```python
from build123d import *

# Parameters (mm, degrees)
SKETCH1_W           = 145
SKETCH1_H           = 85
BOSS_EXTRUDE1_DEPTH = 90
SKETCH3_W           = 130
SKETCH3_H           = 80
CUT_EXTRUDE1_DEPTH  = 85
SKETCH8_R           = 1.7
CUT_EXTRUDE2_DEPTH  = 10
SKETCH9_R           = 1.6
CUT_EXTRUDE3_DEPTH  = 10
SKETCH10_W          = 60.36577322
SKETCH10_H          = 26.383642142
CUT_EXTRUDE4_DEPTH  = 176.87282337
SKETCH11_W          = 127.368574342
SKETCH11_H          = 34.248868694
CUT_EXTRUDE5_DEPTH  = 144.461667354
CUT_EXTRUDE8_DEPTH  = 142
SKETCH13_R          = 2.5
CUT_EXTRUDE9_DEPTH  = 10
FILLET1_R           = 5


with BuildPart() as part:
    # Sketch1 → Boss-Extrude1 (new body)
    with BuildSketch(Plane(origin=(0, 0, 0), x_dir=(1, 0, 0), z_dir=(0, 1, 0))):
        Rectangle(SKETCH1_W, SKETCH1_H)
    extrude(amount=BOSS_EXTRUDE1_DEPTH)

    # Sketch3 → Cut-Extrude1 (cut)
    with BuildSketch(Plane(origin=(0, 90, 0), x_dir=(1, 0, 0), z_dir=(0, 1, 0))):
        Rectangle(SKETCH3_W, SKETCH3_H)
    extrude(amount=-CUT_EXTRUDE1_DEPTH, mode=Mode.SUBTRACT)

    # Sketch8 → Cut-Extrude2 (cut)
    with BuildSketch(Plane(origin=(0, 5, 0), x_dir=(1, 0, 0), z_dir=(0, 1, 0))):
        with Locations(Location((-59.631593059, 20.42, 0), (0, 0, 270))):
            Circle(SKETCH8_R)
        with Locations(Location((-11.231593059, 18.71, 0), (0, 0, 270))):
            Circle(SKETCH8_R)
        with Locations(Location((-54.631593059, -32.1, 0), (0, 0, 270))):
            Circle(SKETCH8_R)
        with Locations(Location((-26.671593059, -32.1, 0), (0, 0, 270))):
            Circle(SKETCH8_R)
    extrude(amount=-CUT_EXTRUDE2_DEPTH, mode=Mode.SUBTRACT)

    # Sketch9 → Cut-Extrude3 (cut)
    with BuildSketch(Plane(origin=(0, 5, 0), x_dir=(1, 0, 0), z_dir=(0, 1, 0))):
        with Locations(Location((57.802096986, 21.3, 0), (0, 0, 270))):
            Circle(SKETCH9_R)
        with Locations(Location((17.802096986, 21.3, 0), (0, 0, 270))):
            Circle(SKETCH9_R)
        with Locations(Location((17.802096986, -18.7, 0), (0, 0, 270))):
            Circle(SKETCH9_R)
        with Locations(Location((57.802096986, -18.7, 0), (0, 0, 270))):
            Circle(SKETCH9_R)
    extrude(amount=-CUT_EXTRUDE3_DEPTH, mode=Mode.SUBTRACT)

    # Sketch10 → Cut-Extrude4 (cut, through all)
    with BuildSketch(Plane(origin=(72.5, 0, 0), x_dir=(0, 0, -1), z_dir=(1, 0, 0))):
        with Locations((0, 36.47748396)):
            Rectangle(SKETCH10_W, SKETCH10_H)
    extrude(amount=-CUT_EXTRUDE4_DEPTH, mode=Mode.SUBTRACT)

    # Sketch11 → Cut-Extrude5 (cut, through all)
    with BuildSketch(Plane(origin=(0, 0, -42.5), x_dir=(-1, 0, 0), z_dir=(0, 0, -1))):
        with Locations((0, 37.630477743)):
            Rectangle(SKETCH11_W, SKETCH11_H)
    extrude(amount=-CUT_EXTRUDE5_DEPTH, mode=Mode.SUBTRACT)

    # Sketch12 → Cut-Extrude8 (cut)
    with BuildSketch(Plane.ZY.offset(72.5)):
        Polygon((-39, 63.608903916), (39, 63.608903916), (39, 74.758903916), (37, 74.758903916), (37, 85.858903916), (-37, 85.858903916), (-37, 74.758903916), (-39, 74.758903916), align=None)
    extrude(amount=-CUT_EXTRUDE8_DEPTH, mode=Mode.SUBTRACT)

    # Sketch13 → Cut-Extrude9 (cut)
    with BuildSketch(Plane.XZ):
        with Locations(Location((46.785911221, -34.286332812, 0), (0, 0, 270))):
            Circle(SKETCH13_R)
        with Locations(Location((0, -34.286332812, 0), (0, 0, 270))):
            Circle(SKETCH13_R)
    extrude(amount=-CUT_EXTRUDE9_DEPTH, mode=Mode.SUBTRACT)

    # Fillet1
    # the kernel refuses this fillet: 5 mm, written as the material it adds along each edge
    with BuildSketch(Plane(origin=(69.5, 87.19624688, -39), x_dir=(-1, 0, 0), z_dir=(0, -1, 0)), Plane(origin=(69.5, 51.171560952, 39), x_dir=(-1, 0, 0), z_dir=(0, 1, 0))) as fillet1_piece_1:
        with BuildLine():
            CenterArc((5, -4.974937186), FILLET1_R, 95.739170477, 84.260829523)
            Line((0, -4.974937186), (-0.1, -4.974937186))
            Line((-0.1, -4.974937186), (-0.1, 0))
            Line((-0.1, 0), (0, 0.1))
            ThreePointArc((0, 0.1), (2.25, 0.1), (4.49, 0.099498744))
            Line((4.49, 0.099498744), (4.5, 0))
        make_face()
    extrude(amount=36.024685928)


solid = part.part
```
For this review, take the finished solid that the model builds, in its own axes (mm). A direction names the side the tool comes from. Round coordinates to 2 decimals unless told otherwise and drop trailing zeros. Write each loop counter-clockwise with the first axis right and the second up, starting at its lowest first coordinate (ties: lowest second). Pieces come first, ordered by that corner, then holes. Notation, with made-up numbers: M -1.5,83.5 L 25.5,83.5 A27 cw 25.5,104.5 Z; hole C -32,-30.5 d7. An arc over 180 degrees is marked long. One line per item, written item: value. Start each with the question number.
(1) We need section A-A (z = 32.1). Give the boundary of the cut face in (x, y).
(2) We need section B-B (x = -37.5). Give the boundary of the cut face in (y, z).
(3) We need section C-C (y = 26.5). Give the boundary of the cut face in (x, z).
(4) The part is to be moulded in two halves that separate along X. For faces 4 (the flat face through (-69, 80, 37)), 5 (the flat face through (-1, 58, -40)), 6 (the flat face through (65, 58, 1)), 7 (the flat face through (-72.5, 14, 1)), say which applies: released by +X, released by -X, zero draft, split by the parting line, or undercut.
(5) Machinability: for faces 1 (the flat face through (-69, 23.286, 0)), 2 (the flat face through (-69, 80, -37)), 3 (the cylindrical face through (-27.706, 2.535, 30.751)), which of the approach directions +Z, -Z, +X, -X, +Y, -Y give a long, thin tool a straight path to every point of the face, cutting with its end or side? Answer none if there is none.
(6) Insertion check: pin 1 (12 mm diameter, centred on y = 76.5, z = -4.5, fed in from -X); pin 2 (2 mm diameter, centred on x = 29.5, z = 9.5, fed in from +Y). Each pin has a flat end and moves straight along its axis. Give the tip position at first contact, or say it passes through.
(7) Wall thickness on line 1 (X direction, y = 3.5, z = 32.1); line 2 (X direction, y = 1.4, z = 18.7); line 3 (X direction, y = 41.5, z = -33.5): over which ranges is each line inside the solid? List them lowest first.
Result:
1. outline: M -72.5,0 L -56.33,0 L -56.33,5 L -65,5 L -65,63.61 L -72.5,63.61 Z; M -72.5,85.86 L -65,85.86 L -65,90 L -72.5,90 Z; M -52.93,0 L -28.37,0 L -28.37,5 L -52.93,5 Z; M -24.97,0 L 72.5,0 L 72.5,90 L 65,90 L 65,85.86 L 69.5,85.86 L 69.5,63.61 L 65,63.61 L 65,5 L -24.97,5 Z
2. outline: M 0,-42.5 L 20.51,-42.5 L 20.51,-40 L 5,-40 L 5,40 L 20.51,40 L 20.51,42.5 L 0,42.5 Z; M 54.75,-42.5 L 90,-42.5 L 90,-40 L 54.75,-40 Z; M 54.75,40 L 90,40 L 90,42.5 L 54.75,42.5 Z
3. outline: M -72.5,-42.5 L -63.68,-42.5 L -63.68,-40 L -65,-40 L -65,-30.18 L -72.5,-30.18 Z; M -72.5,30.18 L -65,30.18 L -65,40 L -63.68,40 L -63.68,42.5 L -72.5,42.5 Z; M 63.68,-42.5 L 72.5,-42.5 L 72.5,-30.18 L 65,-30.18 L 65,-40 L 63.68,-40 Z; M 63.68,40 L 65,40 L 65,30.18 L 72.5,30.18 L 72.5,42.5 L 63.68,42.5 Z
4. face 4: zero draft
4. face 5: undercut
4. face 6: undercut
4. face 7: released by -X
5. face 1: +X, -X
5. face 2: -X
5. face 3: +Y, -Y
6. pin 1: x = 69.5
6. pin 2: y = 5
7. line 1: -72.5 to -56.33, -52.93 to -28.37, -24.97 to 72.5
7. line 2: -72.5 to 16.2, 19.4 to 56.2, 59.4 to 72.5
7. line 3: -72.5 to -65, 65 to 72.5
